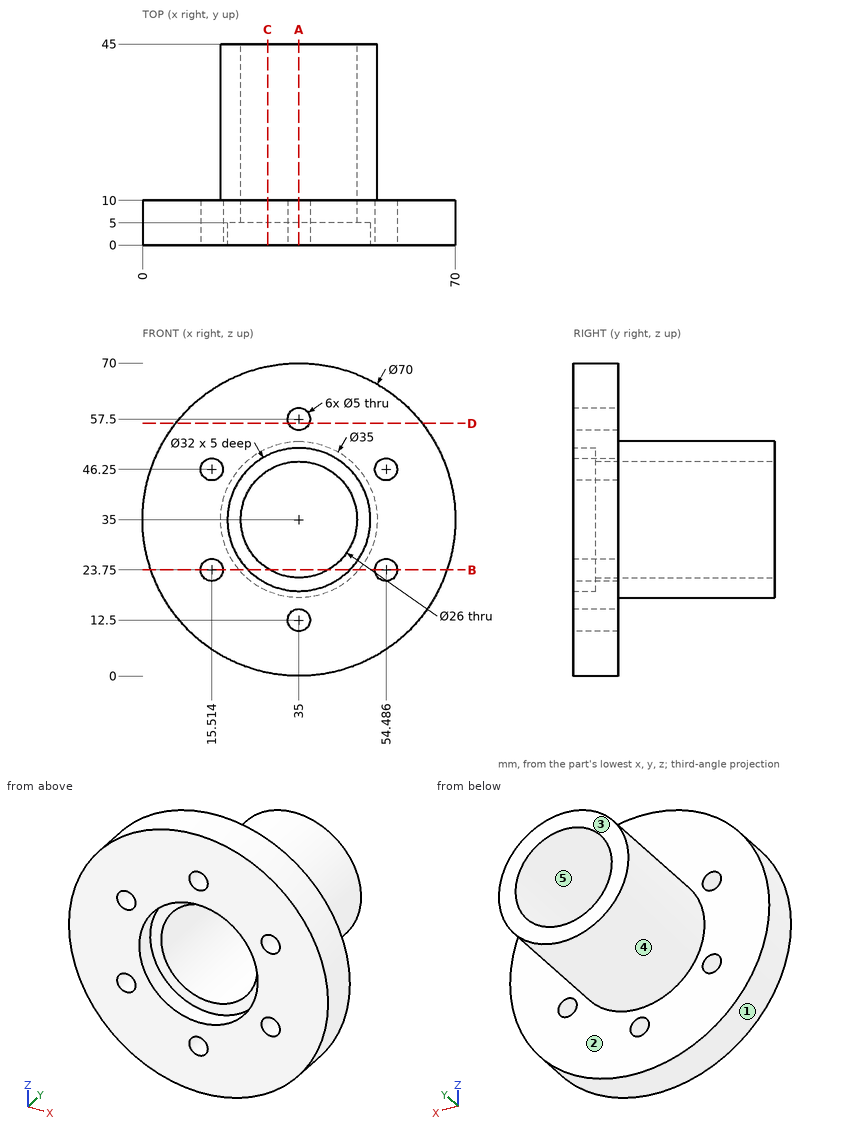
Check sheet for the drawn part. Datum: minimum x, y, z corner. Units: mm. A direction names the side the tool comes from. Give positions to 0.01 mm unless a question says otherwise; leave off trailing zeros. Loops run counter-clockwise (first coordinate to the right, second up) from the corner with the lowest first, then second, coordinate; pieces in that order, holes last. Notation, with made-up numbers: M -11.5,59.25 L 43.5,59.25 A29 cw 43.5,91.25 Z; hole C 64.25,67.25 d9. An arc over 180 degrees is marked long. Return JSON: item names as keys, results as strings.
1) Section check C-C, the plane x = 28. Enter the section's corners in (y, z) (1 decimal).
Findings:
{"outline": "M 0,0.7 L 10,0.7 L 10,19 L 45,19 L 45,24 L 5,24 L 5,20.6 L 0,20.6 Z; M 0,49.4 L 5,49.4 L 5,46 L 45,46 L 45,51 L 10,51 L 10,69.3 L 0,69.3 Z"}
2) Tool access check on the marked faces 1 and 2. Record the directions out of +Z, -Z, +X, -X, +Y, -Y that give a thin tool (end or side, any length) a straight path to the whole face; none if there is none.
Findings:
{"face 1": "+Y, -Y", "face 2": "+Y"}
3) Material ranges on L1, parallel to X at y = 31, z = 35; L2, parallel to Y at x = 23.5, z = 62.5; L3, parallel to X at y = 42, z = 25 (1 decimal), recorded low to high. Write a range as [from, to].
Findings:
{"L1": "x = [17.5, 22], [48, 52.5]", "L2": "y = [0, 10]", "L3": "x = [20.6, 26.7], [43.3, 49.4]"}
4) Mould release check, pull along Z, two halves, no side actions. Record for the marked faces 3, 4 and 5: released by +Z, released by -Z, zero draft, split by the parting line, or undercut.
Findings:
{"face 3": "zero draft", "face 4": "split by the parting line", "face 5": "undercut"}
5) Gauge pin test, flat ends, axial feed: P1, Ø12, axis at y = 37.5, z = 8, coming from the +X side; P2, Ø10, axis at x = 29, y = 33.5, coming from the +Z side; P3, Ø12, axis at x = 62, y = 14, coming from the -Z side (1 decimal); P4, Ø6.5, axis at x = 35, z = 57.5, coming from the +Y side. Record the tip position at first contact, or that the pin passes through.
Findings:
{"P1": "passes through", "P2": "stops at z = 52.47", "P3": "stops at z = 8.2", "P4": "stops at y = 10"}
6) Section check B-B, the plane z = 23.75. Enter the section's corners in (x, y) (1 decimal).
Findings:
{"outline": "M 1.9,0 L 13,0 L 13,10 L 1.9,10 Z; M 18,0 L 23.6,0 L 23.6,5 L 28.5,5 L 28.5,45 L 21.6,45 L 21.6,10 L 18,10 Z; M 41.5,5 L 46.4,5 L 46.4,0 L 52,0 L 52,10 L 48.4,10 L 48.4,45 L 41.5,45 Z; M 57,0 L 68.1,0 L 68.1,10 L 57,10 Z"}
7) Section check D-D, the plane z = 56.5. Enter the section's corners in (x, y).
Findings:
{"outline": "M 7.38,0 L 32.71,0 L 32.71,10 L 7.38,10 Z; M 37.29,0 L 62.62,0 L 62.62,10 L 37.29,10 Z"}
8) Section check A-A, the plane x = 35. Enter the section's corners in (y, z), and give its area (3 significant figures).
Findings:
{"outline": "M 0,0 L 10,0 L 10,10 L 0,10 Z; M 0,15 L 10,15 L 10,17.5 L 45,17.5 L 45,22 L 5,22 L 5,19 L 0,19 Z; M 0,51 L 5,51 L 5,48 L 45,48 L 45,52.5 L 10,52.5 L 10,55 L 0,55 Z; M 0,60 L 10,60 L 10,70 L 0,70 Z", "area": "625 mm2"}
